The model under review builds one solid part; all positions refer to its coordinate system, in mm. A direction names the side the tool comes from. Give positions to 0.01 mm unless a question says otherwise; leave off trailing zeros. Loops run counter-clockwise (first coordinate to the right, second up) from the corner with the lowest first, then second, coordinate; pieces in that order, holes last. Notation, with made-up numbers: M -7,-6 L 47,-6 A27 cw 47,16 Z; hole C 75,0 d3. An arc over 180 degrees is marked long. Return JSON: item names as keys, results as strings. Group by question number.
```python
from build123d import *

# Parameters (mm, degrees)
ESQUISSE1_W             = 20
ESQUISSE1_H             = 20
BOSS_EXTRU_1_DEPTH      = 10
ESQUISSE2_W             = 1.2
ESQUISSE2_H             = 5.5
ESQUISSE2_W_2           = 5.5
ESQUISSE2_H_2           = 1.2
ENL_V_MAT_EXTRU_1_DEPTH = 11
ENL_V_MAT_EXTRU_2_DEPTH = 11
ESQUISSE4_R             = 2.5
ENL_V_MAT_EXTRU_3_DEPTH = 11


with BuildPart() as part:
    # Esquisse1 → Boss.-Extru.1 (new body)
    with BuildSketch(Plane.XY):
        with Locations((-12.505109137, -9.909560068)):
            Rectangle(ESQUISSE1_W, ESQUISSE1_H)
    extrude(amount=BOSS_EXTRU_1_DEPTH)

    # Esquisse2 → Enlèv. mat.-Extru.1 (cut, through all)
    with BuildSketch(Plane.XY.offset(10)):
        with Locations((-21.905109137, -9.909560068)):
            Rectangle(ESQUISSE2_W, ESQUISSE2_H)
        with Locations((-12.505109137, -0.509560068)):
            Rectangle(ESQUISSE2_W_2, ESQUISSE2_H_2)
        with Locations((-3.105109137, -9.909560068)):
            Rectangle(ESQUISSE2_W, ESQUISSE2_H)
        with Locations((-12.505109137, -19.309560068)):
            Rectangle(ESQUISSE2_W_2, ESQUISSE2_H_2)
    extrude(amount=-ENL_V_MAT_EXTRU_1_DEPTH, mode=Mode.SUBTRACT)

    # Esquisse3 → Enlèv. mat.-Extru.2 (cut, through all)
    with BuildSketch(Plane.XY.offset(10)):
        Polygon((-21.305109137, -15.909560068), (-20.305109137, -15.909560068), (-17.305109137, -12.909560068), (-17.305109137, -6.909560068), (-20.305109137, -3.909560068), (-21.305109137, -3.909560068), align=None)
        Polygon((-18.505109137, -1.109560068), (-6.505109137, -1.109560068), (-6.505109137, -2.109560068), (-9.505109137, -5.109560068), (-15.505109137, -5.109560068), (-18.505109137, -2.109560068), align=None)
        Polygon((-3.705109137, -3.909560068), (-4.705109137, -3.909560068), (-7.705109137, -6.909560068), (-7.705109137, -12.909560068), (-4.705109137, -15.909560068), (-3.705109137, -15.909560068), align=None)
        Polygon((-6.505109137, -18.709560068), (-18.505109137, -18.709560068), (-18.505109137, -17.709560068), (-15.505109137, -14.709560068), (-9.505109137, -14.709560068), (-6.505109137, -17.709560068), align=None)
    extrude(amount=-ENL_V_MAT_EXTRU_2_DEPTH, mode=Mode.SUBTRACT)

    # Esquisse4 → Enlèv. mat.-Extru.3 (cut, through all)
    with BuildSketch(Plane.XY.offset(10)):
        with Locations((-12.505109137, -9.909560068)):
            Circle(ESQUISSE4_R)
    extrude(amount=-ENL_V_MAT_EXTRU_3_DEPTH, mode=Mode.SUBTRACT)


solid = part.part
```
(1) For faces 1 (the flat face through (-18.505, -18, 5)), 2 (the flat face through (-9.755, -19, 5)), 3 (the flat face through (-6, -19.91, 5)), list the 3-axis set-ups (+Z, -Z, +X, -X, +Y, -Y) from which the entire face can be reached by the end or side of a thin tool; tool diameter is ignored.
(2) Mouldability with a two-part tool opening along X and no side actions: class faces 4 (the flat face through (-8, -1.11, 5)), 5 (the flat face through (-22, -12.66, 5)), 6 (the flat face through (-7.984, -3.589, 5.07)), 7 (the flat face through (-22.505, -4, 5)) as released by +X, released by -X, zero draft, split by the parting line, or undercut.
(3) Add section B-B (y = -13.75). Write out the cut boundary in (x, z).
(4) For pin 1 (1.8 mm diameter, centred on x = -11.5, z = 2.5, fed in from -Y), flat-tipped, find the tip position at first contact; note if it passes through.
(5) Add section D-D (x = -16.5). Write out the cut boundary in (y, z), and give its area (3 significant figures).
(6) Add section A-A (x = -20.75). Write out the cut boundary in (y, z), and give its area (3 significant figures).
(7) For probe 1 along Y at (x, z) = (-12.5, 1.5); probe 2 along Y at (x, z) = (-7.25, 2.5); probe 3 along X at (y, z) = (-2, 1.5), list the stretches that pass through material, from the lowest coordinate up.
(8) Add section C-C (y = -9). Write out the cut boundary in (x, z).
Verdict:
{
 "1": {"face 1": "+Z, -Z", "face 2": "+Z, -Z, -Y", "face 3": "+Z, -Z, +X, -X, -Y"},
 "2": {"face 4": "undercut", "face 5": "zero draft", "face 6": "undercut", "face 7": "released by -X"},
 "3": {"outline": "M -22.51,0 L -21.31,0 L -21.31,10 L -22.51,10 Z; M -18.15,0 L -6.86,0 L -6.86,10 L -18.15,10 Z; M -3.71,0 L -2.51,0 L -2.51,10 L -3.71,10 Z"},
 "4": {"pin 1": "stops at y = -14.71"},
 "5": {"outline": "M -19.91,0 L -18.71,0 L -18.71,10 L -19.91,10 Z; M -15.7,0 L -4.11,0 L -4.11,10 L -15.7,10 Z; M -1.11,0 L 0.09,0 L 0.09,10 L -1.11,10 Z", "area": "140 mm²"},
 "6": {"outline": "M -19.91,0 L -15.91,0 L -15.91,10 L -19.91,10 Z; M -3.91,0 L 0.09,0 L 0.09,10 L -3.91,10 Z", "area": "80.0 mm²"},
 "7": {"probe 1": "y = -14.71 to -12.41, -7.41 to -5.11", "probe 2": "y = -19.91 to -18.71, -16.96 to -13.36, -6.45 to -2.85, -1.11 to 0.09", "probe 3": "x = -22.51 to -18.51, -6.51 to -2.51"},
 "8": {"outline": "M -17.31,0 L -14.83,0 L -14.83,10 L -17.31,10 Z; M -10.18,0 L -7.71,0 L -7.71,10 L -10.18,10 Z"}
}
